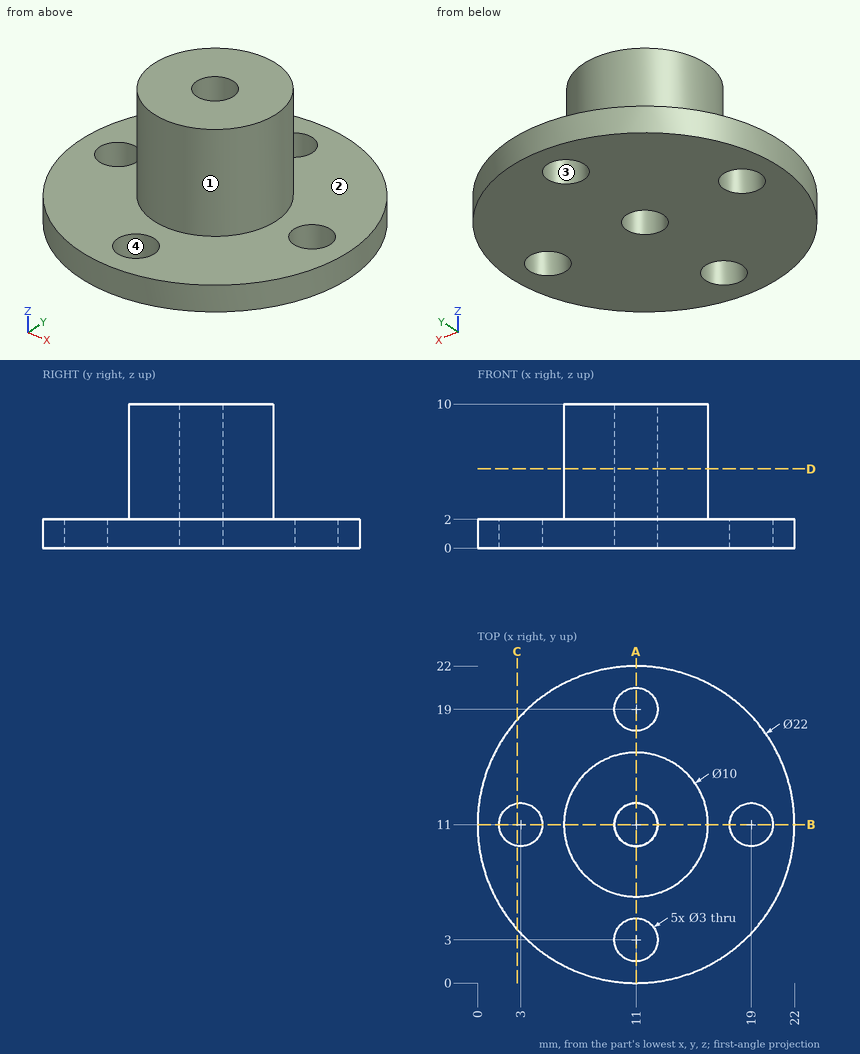
Part print with two shaded views. Sizes in mm from the minimum x, y, z corner. Coordinates: 2 decimals unless noted, no trailing zeros. Write each loop counter-clockwise with the first axis right and the second up, starting at its lowest first coordinate (ties: lowest second). Pieces come first, ordered by that corner, then holes. Notation, with made-up numbers: (27, 70.5) - (81, 70.5) arc R16 cw to (81, 90.5) - close; hole circle Ø9 at (25.5, -21). An arc over 180 degrees is marked (long way). Put each result on its own line as item: value.
1. Band-saw the part on C-C (x = 2.75). Write the cut outline in (y, z).
Final values:
outline: (3.72, 0) - (9.52, 0) - (9.52, 2) - (3.72, 2) - close; (12.48, 0) - (18.28, 0) - (18.28, 2) - (12.48, 2) - close
2. Band-saw the part on D-D (z = 5.5). Write the cut outline in (x, y), then the cut area to 3 significant figures.
Final values:
outline: circle Ø10 at (11, 11); hole circle Ø3 at (11, 11)
area: 71.5 mm²
3. Flat gauge pins, fed straight in: pin 1 Ø3 at (x, z) = (15, 7.5) entering from +Y; pin 2 Ø4 at (x, y) = (11, 3) entering from +Z; pin 3 Ø5 at (y, z) = (19, 1) entering from -X; pin 4 Ø2.5 at (x, y) = (19, 11) entering from -Z. Where does each tip first touch, or does it go through?
Final values:
pin 1: stops at y = 15.33
pin 2: stops at z = 2
pin 3: stops at x = 1.47
pin 4: passes through
4. Probe line 1 along Y through (x, z) = (11, 5.5); line 2 along Z through (x, y) = (18.5, 12.5); line 3 along X through (y, z) = (19.5, 0.75). List the from-to ranges inside material, lowest first. Write a range as [from, to].
Final values:
line 1: y = [6, 9.5], [12.5, 16]
line 2: z = [0, 2]
line 3: x = [4.02, 9.59], [12.41, 17.98]
5. Band-saw the part on A-A (x = 11). Write the cut outline in (y, z).
Final values:
outline: (0, 0) - (1.5, 0) - (1.5, 2) - (0, 2) - close; (4.5, 0) - (9.5, 0) - (9.5, 10) - (6, 10) - (6, 2) - (4.5, 2) - close; (12.5, 0) - (17.5, 0) - (17.5, 2) - (16, 2) - (16, 10) - (12.5, 10) - close; (20.5, 0) - (22, 0) - (22, 2) - (20.5, 2) - close
6. Two-plate mould, pull along X, no slides. Class the marked faces 1, 2, 3 and 4: +X half, -X half, draft (parallel to the pull), parting line (faces both ways), or undercut.
Final values:
face 1: parting line
face 2: draft
face 3: undercut
face 4: undercut
